from build123d import *

# Parameters (mm, degrees)
F0_R     = 25
F0_R_2   = 21
F1_DEPTH = 20
F2_R     = 32.5
F3_DEPTH = 5
F4_R     = 5.5
F5_DEPTH = 5
F6_R     = 10.5
F6_R_2   = 5.5
F7_DEPTH = 20
F9_DEPTH = 20
F10_SIZE = 0.5


with BuildPart() as f1:
    # F0 (on Top) → F1 (new body)
    with BuildSketch(Plane.XY):
        Circle(F0_R)
        Circle(F0_R_2, mode=Mode.SUBTRACT)
    extrude(amount=F1_DEPTH)

    # F2 (on Top) → F3 (join)
    with BuildSketch(Plane.XY):
        Circle(F2_R)
    extrude(amount=-F3_DEPTH)

    # F4 (on face) → F5 (cut, through all)
    with BuildSketch(Plane(origin=(0, 0, -5), x_dir=(1, 0, 0), z_dir=(0, 0, -1))):
        Circle(F4_R)
    extrude(amount=-F5_DEPTH, mode=Mode.SUBTRACT)

    # F6 (on face) → F7 (join)
    with BuildSketch(Plane.XY):
        Circle(F6_R)
        Circle(F6_R_2, mode=Mode.SUBTRACT)
    extrude(amount=F7_DEPTH)

    # F8 (on face) → F9 (join)
    with BuildSketch(Plane.XY):
        with BuildLine():
            Line((-5.5290086594, -8.9263689843), (-8.8208494084, -19.0576130644))
            ThreePointArc((-8.8208494084, -19.0576130644), (-6.4893568819, -19.9721868422), (-4.0655668269, -20.6026980363))
            Line((-4.0655668269, -20.6026980363), (-0.773726078, -10.4714539562))
            ThreePointArc((-0.773726078, -10.4714539562), (-3.2446784409, -9.9860934211), (-5.5290086594, -8.9263689843))
        make_face()
        with BuildLine():
            ThreePointArc((18.3380009794, 10.2331676464), (16.9893568819, 12.3434902981), (15.3990747179, 14.2782526183))
            Line((15.3990747179, 14.2782526183), (6.7809237516, 8.0167994284))
            ThreePointArc((6.7809237516, 8.0167994284), (8.4946784409, 6.1717451491), (9.719850013, 3.9717144565))
            Line((9.719850013, 3.9717144565), (18.3380009794, 10.2331676464))
        make_face()
        with BuildLine():
            Line((6.7809237516, -8.0167994284), (15.3990747179, -14.2782526183))
            ThreePointArc((15.3990747179, -14.2782526183), (16.9893568819, -12.3434902981), (18.3380009794, -10.2331676464))
            Line((18.3380009794, -10.2331676464), (9.719850013, -3.9717144565))
            ThreePointArc((9.719850013, -3.9717144565), (8.4946784409, -6.1717451491), (6.7809237516, -8.0167994284))
        make_face()
        with BuildLine():
            ThreePointArc((-4.0655668269, 20.6026980363), (-6.4893568819, 19.9721868422), (-8.8208494084, 19.0576130644))
            Line((-8.8208494084, 19.0576130644), (-5.5290086594, 8.9263689843))
            ThreePointArc((-5.5290086594, 8.9263689843), (-3.2446784409, 9.9860934211), (-0.773726078, 10.4714539562))
            Line((-0.773726078, 10.4714539562), (-4.0655668269, 20.6026980363))
        make_face()
        with BuildLine():
            Line((-10.1980390272, 2.5), (-20.850659462, 2.5))
            ThreePointArc((-20.850659462, 2.5), (-21, 0), (-20.850659462, -2.5))
            Line((-20.850659462, -2.5), (-10.1980390272, -2.5))
            ThreePointArc((-10.1980390272, -2.5), (-10.5, 0), (-10.1980390272, 2.5))
        make_face()
    extrude(amount=F9_DEPTH)

    # F10
    f10_edges = [f1.edges().sort_by_distance(p)[0] for p in [
        (25, 0, 10),
        (-25, 0, 0),
        (-25, 0, 20),
    ]]
    chamfer(f10_edges, length=F10_SIZE)


solid = f1.part
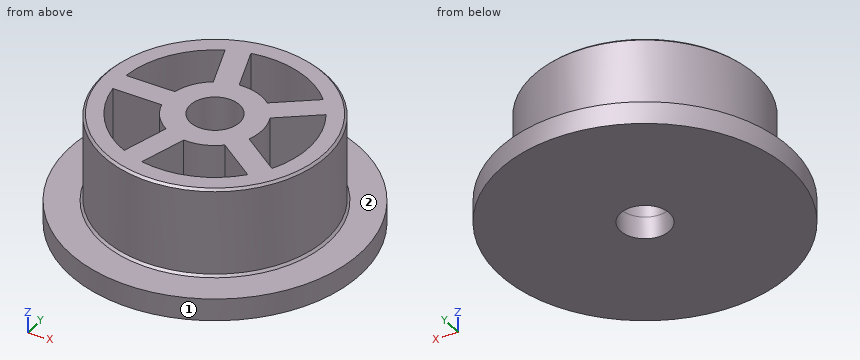
Input: part model. Units: mm. Frame: model coordinates. Face numbers are marked on the shaded views. A direction names the side the tool comes from. Give positions to 0.01 mm unless a question says otherwise; leave off trailing zeros. Write each loop counter-clockwise with the first axis right and the second up, starting at its lowest first coordinate (ties: lowest second). Pieces come first, ordered by that corner, then holes. Notation, with made-up numbers: M -30,-28 L 4,-28 A23 cw 4,-8 Z; hole C 37.5,86.5 d4. An arc over 180 degrees is marked long. Write item = value, one per line. Start each with the question number.
1) Cut plane A-A on z = 2.5. Return the cut outline in (x, y).
2) Cut plane D-D on z = -1.5. Return the cut outline in (x, y).
3) Reachability of the marked faces 1 and 2 from +Z, -Z, +X, -X, +Y, -Y: full face, straight path, thin tool, end or side. Return the list, or none.
4) First-contact query: pin 1 Ø17.5 at (x, y) = (0, 0) entering from -Z; pin 2 Ø6.5 at (x, y) = (8.5, -13.5) entering from +Z; pin 3 Ø10 at (x, z) = (17.5, 5.5) entering from -Y; pin 4 Ø8.5 at (x, z) = (-14.5, 8.5) entering from -Y. Flat tips, straight axial feed; report the tip coordinate or a pass-through.
5) Cut plane C-C on y = 0. Return the cut outline in (x, z).
6) Cut plane B-B on x = 0. Return the cut outline in (y, z).
7) Material intervals for line 1 along Y through (x, z) = (0, 6.5); line 2 along X through (y, z) = (16, 3); line 3 along Y through (x, z) = (13, 11.5), sorted ascending. Write a range as [from, to].
Solved:
q1.outline = C 0,0 d50; hole M -20.85,-2.5 A21 ccw -8.82,-19.06 L -5.53,-8.93 A10.5 cw -10.2,-2.5 Z; hole M -20.85,2.5 L -10.2,2.5 A10.5 cw -5.53,8.93 L -8.82,19.06 A21 ccw Z; hole C 0,0 d11; hole M -4.07,-20.6 A21 ccw 15.4,-14.28 L 6.78,-8.02 A10.5 cw -0.77,-10.47 Z; hole M -4.07,20.6 L -0.77,10.47 A10.5 cw 6.78,8.02 L 15.4,14.28 A21 ccw Z; hole M 9.72,-3.97 L 18.34,-10.23 A21 ccw 18.34,10.23 L 9.72,3.97 A10.5 cw Z
q2.outline = C 0,0 d65; hole C 0,0 d11
q3.face_1 = +Z, -Z
q3.face_2 = +Z
q4.pin_1 = -5
q4.pin_2 = 0
q4.pin_3 = -21.65
q4.pin_4 = -22.8
q5.outline = M -32.5,-5 L -5.5,-5 L -5.5,20 L -24.5,20 L -25,19.5 L -25,0.5 L -25.5,0 L -32.5,0 Z; M 5.5,-5 L 32.5,-5 L 32.5,0 L 25.5,0 L 25,0.5 L 25,19.5 L 24.5,20 L 21,20 L 21,0 L 10.5,0 L 10.5,20 L 5.5,20 Z
q6.outline = M -32.5,-5 L -5.5,-5 L -5.5,20 L -10.5,20 L -10.5,0 L -21,0 L -21,20 L -24.5,20 L -25,19.5 L -25,0.5 L -25.5,0 L -32.5,0 Z; M 5.5,-5 L 32.5,-5 L 32.5,0 L 25.5,0 L 25,0.5 L 25,19.5 L 24.5,20 L 21,20 L 21,0 L 10.5,0 L 10.5,20 L 5.5,20 Z
q7.line_1 = [-25, -21], [-10.5, -5.5], [5.5, 10.5], [21, 25]
q7.line_2 = [-19.21, -13.6], [-7.83, -2.57], [13.6, 19.21]
q7.line_3 = [-21.35, -16.49], [-12.54, -6.35], [6.35, 12.54], [16.49, 21.35]
